Autodesk Inventor part; units mm, degrees
ref_plane "YZ Plane" through (0, 0, 0) normal (1, 0, 0) x (0, 1, 0)
ref_plane "XZ Plane" through (0, 0, 0) normal (0, 1, 0) x (-1, 0, 0)
ref_plane "XY Plane" through (0, 0, 0) normal (0, 0, 1) x (1, 0, 0)
ref_plane "Work Plane1" through (0, 0, 0) normal (0, 0, 1) x (1, 0, 0)
sketch "Sketch1" plane through (0, 0, 0) normal (0, 0, 1) x (1, 0, 0)
  line L0 (35.585, -35.585) -> (35.585, 35.585)
  line L1 (-35.585, -35.585) -> (35.585, -35.585)
  line L2 (35.615, -35.585) -> (106.785, -35.585)
  line L3 (35.615, -35.615) -> (35.615, -106.785)
  line L4 (-35.585, 35.585) -> (-35.585, -35.585)
  line L5 (35.585, 35.585) -> (-35.585, 35.585)
  line L6 (106.785, 35.585) -> (35.615, 35.585)
  line L7 (106.785, -35.585) -> (106.785, 35.585)
  line L8 (35.585, -35.585) -> (35.615, -35.615)
  line L9 (35.615, -35.585) -> (35.585, -35.615)
  line L10 (35.585, 35.8807) -> (107.085, 35.8807) construction
  line L11 (-35.915, 35.8807) -> (-35.915, 36.8807)
  line L12 (104.585, 37.3807) -> (-33.415, 37.3807)
  line L13 (-37.415, 33.3807) -> (-37.415, -104.6193)
  line L14 (-33.415, -108.6193) -> (104.585, -108.6193)
  line L15 (108.585, -104.6193) -> (108.585, 33.3807)
  arc A0 (104.585, -108.6193) -> (108.585, -104.6193) centre (104.585, -104.6193) ccw
  arc A1 (-37.415, -104.6193) -> (-33.415, -108.6193) centre (-33.415, -104.6193) ccw
  arc A2 (-33.415, 37.3807) -> (-37.415, 33.3807) centre (-33.415, 33.3807) ccw
  arc A3 (108.585, 33.3807) -> (104.585, 37.3807) centre (104.585, 33.3807) ccw
  line L16 (35.6, 49.4) -> (-39.4, 49.4)
  line L17 (120.6, 39.4) -> (120.6, -110.6)
  line L18 (110.6, -120.6) -> (-39.4, -120.6)
  line L19 (-49.4, -110.6) -> (-49.4, 39.4)
  arc A4 (-39.4, 49.4) -> (-49.4, 39.4) centre (-39.4, 39.4) ccw
  arc A5 (120.6, 39.4) -> (110.6, 49.4) centre (110.6, 39.4) ccw
  arc A6 (110.6, -120.6) -> (120.6, -110.6) centre (110.6, -110.6) ccw
  arc A7 (-49.4, -110.6) -> (-39.4, -120.6) centre (-39.4, -110.6) ccw
  line L20 (35.6, 49.4) -> (110.6, 49.4)
  point P0 (0, 0)
  point P1 (120.6, -120.6)
  point P2 (120.6, 49.4)
  point P3 (-49.4, -120.6)
  dimension "d2" = 71.5
  dimension "d15" = 1
  dimension "d18" = 4
  dimension "d21" = 170
  dimension "d22" = 170
  dimension "d23" = 10
extrude "Extrusion2" add sketch "Sketch1" against normal blind 10 contours L20 A5 L17 A6 L18 A7 L19 A4 L16
sketch "Sketch3" plane through (0, 0, 0) normal (0, 0, 1) x (1, 0, 0)
  arc A0 (104.585, -108.6193) -> (108.585, -104.6193) centre (104.585, -104.6193) ccw
  line L0 (104.585, -108.6193) -> (-33.415, -108.6193)
  arc A1 (-37.415, -104.6193) -> (-33.415, -108.6193) centre (-33.415, -104.6193) ccw
  line L1 (-37.415, -104.6193) -> (-37.415, 33.3807)
  arc A2 (-33.415, 37.3807) -> (-37.415, 33.3807) centre (-33.415, 33.3807) ccw
  line L2 (-33.415, 37.3807) -> (104.585, 37.3807)
  arc A3 (108.585, 33.3807) -> (104.585, 37.3807) centre (104.585, 33.3807) ccw
  line L3 (108.585, 33.3807) -> (108.585, -104.6193)
  line L4 (110.6, 49.4) -> (-39.4, 49.4)
  arc A4 (-39.4, 49.4) -> (-49.4, 39.4) centre (-39.4, 39.4) ccw
  line L5 (-49.4, 39.4) -> (-49.4, -110.6)
  arc A5 (-49.4, -110.6) -> (-39.4, -120.6) centre (-39.4, -110.6) ccw
  line L6 (-39.4, -120.6) -> (110.6, -120.6)
  arc A6 (110.6, -120.6) -> (120.6, -110.6) centre (110.6, -110.6) ccw
  line L7 (120.6, -110.6) -> (120.6, 39.4)
  arc A7 (120.6, 39.4) -> (110.6, 49.4) centre (110.6, 39.4) ccw
  line L8 (108.585, -93.6) -> (-37.415, -93.6)
  line L9 (-37.415, -48.6) -> (108.585, -48.6)
  line L10 (108.585, 22.4) -> (-37.415, 22.4)
  line L11 (-37.415, -22.6) -> (108.585, -22.6)
  line L12 (108.585, 22.4) -> (108.585, -22.6)
  line L13 (-37.415, 22.4) -> (-37.415, -22.6)
  line L14 (-37.415, -48.6) -> (-37.415, -93.6)
  line L15 (108.585, -48.6) -> (108.585, -93.6)
  point P0 (0, 0)
  dimension "d27" = 45
extrude "Extrusion3" add sketch "Sketch3" along normal blind 20 contours L8 L1 L9 L3 | L11 L1 L10 L3 | A7 L7 A6 L6 A5 L5 A4 L4
sketch "Sketch5" plane through (0, 0, -10) normal (0, 0, -1) x (-1, 0, 0)
  arc A0 (-108.585, -104.6193) -> (-104.585, -108.6193) centre (-104.585, -104.6193) ccw
  line L0 (-108.585, -104.6193) -> (-108.585, 33.3807)
  arc A1 (-104.585, 37.3807) -> (-108.585, 33.3807) centre (-104.585, 33.3807) ccw
  line L1 (-104.585, 37.3807) -> (33.415, 37.3807)
  arc A2 (37.415, 33.3807) -> (33.415, 37.3807) centre (33.415, 33.3807) ccw
  line L2 (37.415, 33.3807) -> (37.415, -104.6193)
  arc A3 (33.415, -108.6193) -> (37.415, -104.6193) centre (33.415, -104.6193) ccw
  line L3 (33.415, -108.6193) -> (-104.585, -108.6193)
  line L4 (33.415, 41.3807) -> (-104.585, 41.3807)
  arc A4 (-104.585, 41.3807) -> (-112.585, 33.3807) centre (-104.585, 33.3807) ccw
  line L5 (-112.585, 33.3807) -> (-112.585, -104.6193)
  arc A5 (-112.585, -104.6193) -> (-104.585, -112.6193) centre (-104.585, -104.6193) ccw
  line L6 (-104.585, -112.6193) -> (33.415, -112.6193)
  arc A6 (33.415, -112.6193) -> (41.415, -104.6193) centre (33.415, -104.6193) ccw
  line L7 (41.415, -104.6193) -> (41.415, 33.3807)
  arc A7 (41.415, 33.3807) -> (33.415, 41.3807) centre (33.415, 33.3807) ccw
  point P0 (0, 0)
  dimension "d32" = 4
extrude "Extrusion5" cut sketch "Sketch5" against normal blind 3
sketch "Sketch6" plane through (0, 0, -10) normal (0, 0, -1) x (-1, 0, 0)
  line L0 (39.4, 49.4) -> (-110.6, 49.4)
  arc A0 (-110.6, 49.4) -> (-120.6, 39.4) centre (-110.6, 39.4) ccw
  line L1 (-120.6, 39.4) -> (-120.6, -110.6)
  arc A1 (-120.6, -110.6) -> (-110.6, -120.6) centre (-110.6, -110.6) ccw
  line L2 (-110.6, -120.6) -> (39.4, -120.6)
  arc A2 (39.4, -120.6) -> (49.4, -110.6) centre (39.4, -110.6) ccw
  line L3 (49.4, -110.6) -> (49.4, 39.4)
  arc A3 (49.4, 39.4) -> (39.4, 49.4) centre (39.4, 39.4) ccw
  line L4 (-110.6, 45.4) -> (39.4, 45.4)
  arc A4 (45.4, 39.4) -> (39.4, 45.4) centre (39.4, 39.4) ccw
  line L5 (45.4, 39.4) -> (45.4, -110.6)
  arc A5 (39.4, -116.6) -> (45.4, -110.6) centre (39.4, -110.6) ccw
  line L6 (39.4, -116.6) -> (-110.6, -116.6)
  arc A6 (-116.6, -110.6) -> (-110.6, -116.6) centre (-110.6, -110.6) ccw
  line L7 (-116.6, -110.6) -> (-116.6, 39.4)
  arc A7 (-110.6, 45.4) -> (-116.6, 39.4) centre (-110.6, 39.4) ccw
  point P0 (0, 0)
  dimension "d35" = 4
extrude "Extrusion6" cut sketch "Sketch6" against normal blind 15
sketch "Sketch7" plane through (0, 0, 20) normal (0, 0, 1) x (1, 0, 0)
  line L0 (110.6, 49.4) -> (-39.4, 49.4)
  arc A0 (-39.4, 49.4) -> (-49.4, 39.4) centre (-39.4, 39.4) ccw
  line L1 (-49.4, 39.4) -> (-49.4, -110.6)
  arc A1 (-49.4, -110.6) -> (-39.4, -120.6) centre (-39.4, -110.6) ccw
  line L2 (-39.4, -120.6) -> (110.6, -120.6)
  arc A2 (110.6, -120.6) -> (120.6, -110.6) centre (110.6, -110.6) ccw
  line L3 (120.6, -110.6) -> (120.6, 39.4)
  arc A3 (120.6, 39.4) -> (110.6, 49.4) centre (110.6, 39.4) ccw
  line L4 (-39.4, 45.4) -> (110.6, 45.4)
  arc A4 (116.6, 39.4) -> (110.6, 45.4) centre (110.6, 39.4) ccw
  line L5 (116.6, 39.4) -> (116.6, -110.6)
  arc A5 (110.6, -116.6) -> (116.6, -110.6) centre (110.6, -110.6) ccw
  line L6 (110.6, -116.6) -> (-39.4, -116.6)
  arc A6 (-45.4, -110.6) -> (-39.4, -116.6) centre (-39.4, -110.6) ccw
  line L7 (-45.4, -110.6) -> (-45.4, 39.4)
  arc A7 (-39.4, 45.4) -> (-45.4, 39.4) centre (-39.4, 39.4) ccw
  point P0 (0, 0)
  dimension "d38" = 4
extrude "Extrusion7" cut sketch "Sketch7" against normal blind 10
properties part number "Case" material "Aluminum 6061"
Build history of the part. All positions in model axes, mm. A direction names the side the tool comes from. Coordinates: 2 decimals unless noted, no trailing zeros. Order: outer loops, then holes, each group sorted by start corner. A loop starts at its lowest first (then second) coordinate and runs counter-clockwise, first axis right, second up.
Item 1: Drill centre lines: L1, parallel to Y at x = 13.5, z = 13; L2, parallel to Y at x = 6.5, z = 8; L3, parallel to X at y = -46, z = 11.25 (3 decimals). Where is each one in solid material? Low to high.
Filled in:
L1: y = -116.6 to -108.62, -93.6 to -48.6, -22.6 to 22.4, 37.38 to 45.4
L2: y = -120.6 to -108.62, -93.6 to -48.6, -22.6 to 22.4, 37.38 to 49.4
L3: x = -45.4 to -37.415, 108.585 to 116.6
Item 2: Saw through at B-B on y = -40. List the corners of the cut face in (x, z) (3 decimals), then the cut area to 3 significant figures.
Filled in:
outline: (-49.4, 5) - (-45.4, 5) - (-45.4, -10) - (-41.415, -10) - (-41.415, -7) - (-37.415, -7) - (-37.415, 20) - (-45.4, 20) - (-45.4, 10) - (-49.4, 10) - close; (108.585, -7) - (112.585, -7) - (112.585, -10) - (116.6, -10) - (116.6, 5) - (120.6, 5) - (120.6, 10) - (116.6, 10) - (116.6, 20) - (108.585, 20) - close
area: 496 mm2
Item 3: Saw through at A-A on x = 87.5. List the corners of the cut face in (y, z).
Filled in:
outline: (-120.6, 5) - (-116.6, 5) - (-116.6, -10) - (-112.62, -10) - (-112.62, -7) - (-108.62, -7) - (-108.62, 20) - (-116.6, 20) - (-116.6, 10) - (-120.6, 10) - close; (-93.6, 0) - (-48.6, 0) - (-48.6, 20) - (-93.6, 20) - close; (-22.6, 0) - (22.4, 0) - (22.4, 20) - (-22.6, 20) - close; (37.38, -7) - (41.38, -7) - (41.38, -10) - (45.4, -10) - (45.4, 5) - (49.4, 5) - (49.4, 10) - (45.4, 10) - (45.4, 20) - (37.38, 20) - close
Item 4: Drop flat-ended pins along their axis: pin 1 Ø4 at (y, z) = (-61, 10.5) entering from +X; pin 2 Ø2 at (x, z) = (8.5, -1.5) entering from +Y; pin 3 Ø12 at (y, z) = (0.5, -3.5) entering from -X; pin 4 Ø2 at (y, z) = (-18, -4) entering from +X. Give the stop position or say it passes through.
Filled in:
pin 1: stops at x = 120.6
pin 2: stops at y = 45.4
pin 3: stops at x = -45.4
pin 4: stops at x = 116.6
Item 5: Saw through at D-D on z = -4.25. List the corners of the cut face in (x, y) (3 decimals), then the cut area to 3 significant figures.
Filled in:
outline: (-45.4, -110.6) arc R6 ccw to (-39.4, -116.6) - (110.6, -116.6) arc R6 ccw to (116.6, -110.6) - (116.6, 39.4) arc R6 ccw to (110.6, 45.4) - (-39.4, 45.4) arc R6 ccw to (-45.4, 39.4) - close; hole (-37.415, -104.619) arc R4 ccw to (-33.415, -108.619) - (104.585, -108.619) arc R4 ccw to (108.585, -104.619) - (108.585, 33.381) arc R4 ccw to (104.585, 37.381) - (-33.415, 37.381) arc R4 ccw to (-37.415, 33.381) - close
area: 4,910 mm2
Item 6: Mould opens along X. For faces 6 (the flat face through (36, -117, 5)), 7 (the flat face through (108.585, -37, 4)), 8 (the flat face through (-45.4, -35, -3)), 9 (the flat face through (35, -48.6, 10)) say: released by +X, released by -X, zero draft, split by the parting line, or undercut.
Filled in:
face 6: zero draft
face 7: undercut
face 8: released by -X
face 9: undercut
Item 7: Saw through at C-C on z = 12.5. List the corners of the cut face in (x, y) (3 decimals).
Filled in:
outline: (-45.4, -110.6) arc R6 ccw to (-39.4, -116.6) - (110.6, -116.6) arc R6 ccw to (116.6, -110.6) - (116.6, 39.4) arc R6 ccw to (110.6, 45.4) - (-39.4, 45.4) arc R6 ccw to (-45.4, 39.4) - close; hole (-37.415, -104.619) arc R4 ccw to (-33.415, -108.619) - (104.585, -108.619) arc R4 ccw to (108.585, -104.619) - (108.585, -93.6) - (-37.415, -93.6) - close; hole (-37.415, -48.6) - (108.585, -48.6) - (108.585, -22.6) - (-37.415, -22.6) - close; hole (-37.415, 22.4) - (108.585, 22.4) - (108.585, 33.381) arc R4 ccw to (104.585, 37.381) - (-33.415, 37.381) arc R4 ccw to (-37.415, 33.381) - close
Item 8: Tool access for faces 1 (the flat face through (35, 0, 0)), 2 (the flat face through (116.6, -37, -3)), 3 (the cylindrical face through (114.889, -114.796, -2.605)), 4 (the cylindrical face through (-43.689, 43.596, -2.605)), 5 (the flat face through (37, 37.381, 7)): list every direction of +Z, -Z, +X, -X, +Y, -Y with a clear straight run to the whole face (end or side of a thin tool).
Filled in:
face 1: -Z
face 2: -Z, +X, +Y, -Y
face 3: -Z, +X, -Y
face 4: -Z, -X, +Y
face 5: +Z, -Z
